Work out the finished part from the listing and answer in its coordinate system (mm). Coordinates: 2 decimals unless noted, no trailing zeros. Order: outer loops, then holes, each group sorted by start corner. A loop starts at its lowest first (then second) coordinate and runs counter-clockwise, first axis right, second up. Notation, with made-up numbers: M -12.75,-36.5 L 35.25,-36.5 A22 cw 35.25,1.5 Z; hole C 10.25,12 d6. An arc over 180 degrees is marked long. Answer in a Markdown table with one row per item. Add a question column.
Item 1: Consider line 1 (Z direction, x = 127.5, y = 1.75); line 2 (X direction, y = 3.9, z = 13); line 3 (Z direction, x = 57, y = 4.55). Determine where each line is inside the solid, lowest interval first. Write a range as from..to.
Item 2: The part is cut by section C-C (z = 33). Write down the section's boundary in (x, y), then the cut area to 3 significant figures.
Item 3: The part is cut by section A-A (z = 7). Write down the section's boundary in (x, y), then the cut area to 3 significant figures.
Item 4: The part is cut by section D-D (x = 19). Write down the section's boundary in (y, z), then the cut area to 3 significant figures.
Item 5: The part is cut by section B-B (x = 51). Write down the section's boundary in (y, z).
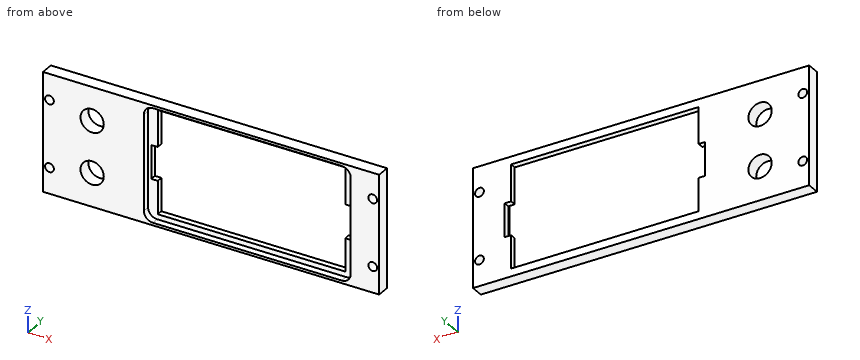
Autodesk Fusion 360 part; units mm, degrees
sketch "Sketch1" plane through (0, 0, 0) normal (0, 0, 1) x (1, 0, 0)
  line L0 (0, 0) -> (130, 0)
  line L1 (130, 0) -> (130, 5)
  line L2 (130, 5) -> (0, 5)
  line L3 (0, 5) -> (0, 0)
  dimension "d1" = 130
  dimension "d2" = 5
extrude "Extrude1" add sketch "Sketch1" along normal blind 46
sketch "Sketch2" plane through (0, 0, 0) normal (0, -1, 0) x (1, 0, 0)
  line L0 (0, 0) -> (130, 0)
  line L1 (130, 0) -> (130, 46)
  line L2 (130, 46) -> (0, 46)
  line L3 (0, 46) -> (0, 0)
  line L4 (42.5, 45) -> (115.5, 45)
  line L5 (119, 41.5) -> (119, 4.5)
  line L6 (115.5, 1) -> (42.5, 1)
  line L7 (39, 4.5) -> (39, 41.5)
  line L8 (125, 46) -> (125, 0) construction
  line L9 (5, 46) -> (5, 0) construction
  line L10 (42.75, 43) -> (115.25, 43)
  line L11 (115.25, 3) -> (42.75, 3)
  line L12 (42.75, 28.8154) -> (40.25, 28.8154)
  line L13 (40.25, 28.8154) -> (40.25, 15.8154)
  line L14 (40.25, 15.8154) -> (42.75, 15.8154)
  line L15 (115.25, 28.8154) -> (117.75, 28.8154)
  line L16 (117.75, 28.8154) -> (117.75, 15.8154)
  line L17 (117.75, 15.8154) -> (115.25, 15.8154)
  line L18 (115.25, 43) -> (115.25, 28.8154)
  line L19 (115.25, 15.8154) -> (115.25, 3)
  line L20 (42.75, 3) -> (42.75, 15.8154)
  line L21 (42.75, 28.8154) -> (42.75, 43)
  arc A0 (42.5, 45) -> (39, 41.5) centre (42.5, 41.5) ccw
  arc A1 (119, 41.5) -> (115.5, 45) centre (115.5, 41.5) ccw
  arc A2 (115.5, 1) -> (119, 4.5) centre (115.5, 4.5) ccw
  arc A3 (39, 4.5) -> (42.5, 1) centre (42.5, 4.5) ccw
  point P0 (39, 45)
  point P1 (119, 45)
  point P2 (39, 1)
  dimension "d5" = 80
  dimension "d6" = 44
  dimension "d7" = 5
  dimension "d8" = 5
  dimension "d9" = 6
  dimension "d10" = 1
  dimension "d25" = 2.5
  dimension "d26" = 13
  dimension "d28" = 13
  dimension "d35" = 3.5
  dimension "d59" = 72.5
  dimension "d60" = 40
  dimension "d62" = 2.5
  dimension "d63" = 1.25
  dimension "d64" = 2
extrude "Extrude5" cut sketch "Sketch2" against normal blind 5 contours L10 L11 L12 L13 L14 L15 L16 L17 L18 L19 L20 L21
sketch "Sketch4" plane through (0, 5, 0) normal (0, 1, 0) x (-1, 0, 0)
  line L0 (-40.25, 15.8154) -> (-42.75, 15.8154)
  line L1 (-42.75, 15.8154) -> (-42.75, 3)
  line L2 (-42.75, 3) -> (-115.25, 3)
  line L3 (-115.25, 3) -> (-115.25, 15.8154)
  line L4 (-115.25, 15.8154) -> (-117.75, 15.8154)
  line L5 (-117.75, 15.8154) -> (-117.75, 28.8154)
  line L6 (-117.75, 28.8154) -> (-115.25, 28.8154)
  line L7 (-115.25, 28.8154) -> (-115.25, 43)
  line L8 (-115.25, 43) -> (-42.75, 43)
  line L9 (-42.75, 43) -> (-42.75, 28.8154)
  line L10 (-42.75, 28.8154) -> (-40.25, 28.8154)
  line L11 (-40.25, 28.8154) -> (-40.25, 15.8154)
  line L12 (-130, 0) -> (0, 0)
  line L13 (0, 0) -> (0, 46)
  line L14 (0, 46) -> (-130, 46)
  line L15 (-130, 46) -> (-130, 0)
  line L16 (-118.25, 45) -> (-39.25, 45)
  line L17 (-39.25, 45) -> (-39.25, 2)
  line L18 (-39.25, 2) -> (-118.25, 2)
  line L19 (-118.25, 2) -> (-118.25, 45)
  line L20 (-42.75, 43) -> (-115.25, 43)
  dimension "d31" = 79
  dimension "d32" = 43
  dimension "d33" = 2
  dimension "d34" = 3.5
extrude "Extrude6" cut sketch "Sketch2" against normal blind 2.7 contours L4 L5 L6 L7 A0 A1 A2 A3
sketch "Sketch5" plane through (0, 0, 0) normal (0, -1, 0) x (1, 0, 0)
  line L0 (39, 4.5) -> (39, 41.5)
  arc A0 (42.5, 45) -> (39, 41.5) centre (42.5, 41.5) ccw
  line L1 (42.5, 45) -> (115.5, 45)
  arc A1 (119, 41.5) -> (115.5, 45) centre (115.5, 41.5) ccw
  line L2 (119, 41.5) -> (119, 4.5)
  arc A2 (115.5, 1) -> (119, 4.5) centre (115.5, 4.5) ccw
  line L3 (115.5, 1) -> (42.5, 1)
  arc A3 (39, 4.5) -> (42.5, 1) centre (42.5, 4.5) ccw
  line L4 (0, 0) -> (130, 0)
  line L5 (130, 0) -> (130, 46)
  line L6 (130, 46) -> (0, 46)
  line L7 (0, 46) -> (0, 0)
  line L8 (19, 33) -> (19, 13) construction
  line L9 (5, 46) -> (5, 0) construction
  line L10 (39, 23) -> (19, 23) construction
  point P0 (19, 33)
  point P1 (19, 13)
  point P2 (19, 33)
  point P3 (19, 33)
  point P4 (19, 33)
  point P5 (19, 13)
  dimension "d40" = 20
  dimension "d41" = 20
  dimension "d42" = 5
hole "Hole1" at (19, 0, 33) at (19, 0, 13) direction (0, 1, 0) diameter 9 end through all
sketch "Sketch6" plane through (0, 0, 0) normal (0, -1, 0) x (1, 0, 0)
  circle A0 centre (19, 33) radius 4.5
  circle A1 centre (19, 13) radius 4.5
  line L0 (39, 4.5) -> (39, 41.5)
  arc A2 (42.5, 45) -> (39, 41.5) centre (42.5, 41.5) ccw
  line L1 (42.5, 45) -> (115.5, 45)
  arc A3 (119, 41.5) -> (115.5, 45) centre (115.5, 41.5) ccw
  line L2 (119, 41.5) -> (119, 4.5)
  arc A4 (115.5, 1) -> (119, 4.5) centre (115.5, 4.5) ccw
  line L3 (115.5, 1) -> (42.5, 1)
  arc A5 (39, 4.5) -> (42.5, 1) centre (42.5, 4.5) ccw
  line L4 (0, 0) -> (130, 0)
  line L5 (130, 0) -> (130, 46)
  line L6 (130, 46) -> (0, 46)
  line L7 (0, 46) -> (0, 0)
  line L8 (125, 46) -> (125, 0) construction
  line L9 (5, 46) -> (5, 0) construction
  point P0 (2.5, 36)
  point P1 (2.5, 10)
  point P2 (127.5, 36)
  point P3 (127.5, 10)
  dimension "d46" = 5
  dimension "d47" = 5
  dimension "d48" = 2.5
  dimension "d49" = 10
  dimension "d50" = 10
  dimension "d51" = 2.5
  dimension "d52" = 2.5
  dimension "d53" = 10
  dimension "d54" = 10
  dimension "d55" = 2.5
hole "Hole2" at (127.5, 0, 36) at (127.5, 0, 10) at (2.5, 0, 36) at (2.5, 0, 10) direction (0, 1, 0) diameter 3.4 depth 5 tip angle 180
Reply:
| question | item | result |
|---|---|---|
| 1 | line 1 | z = 0..8.3, 11.7..34.3, 37.7..46 |
| 1 | line 2 | x = 0..14.5, 23.5..42.75, 115.25..130 |
| 1 | line 3 | z = 0..3, 43..46 |
| 2 | outline | M 0,0 L 14.5,0 L 14.5,5 L 0,5 Z; M 23.5,0 L 39,0 L 39,2.7 L 42.75,2.7 L 42.75,5 L 23.5,5 Z; M 115.25,2.7 L 119,2.7 L 119,0 L 130,0 L 130,5 L 115.25,5 Z |
| 2 | area | 222 mm2 |
| 3 | outline | M 0,0 L 39,0 L 39,2.7 L 42.75,2.7 L 42.75,5 L 0,5 Z; M 115.25,2.7 L 119,2.7 L 119,0 L 130,0 L 130,5 L 115.25,5 Z |
| 3 | area | 267 mm2 |
| 4 | outline | M 0,0 L 5,0 L 5,8.5 L 0,8.5 Z; M 0,17.5 L 5,17.5 L 5,28.5 L 0,28.5 Z; M 0,37.5 L 5,37.5 L 5,46 L 0,46 Z |
| 4 | area | 140 mm2 |
| 5 | outline | M 0,0 L 5,0 L 5,3 L 2.7,3 L 2.7,1 L 0,1 Z; M 0,45 L 2.7,45 L 2.7,43 L 5,43 L 5,46 L 0,46 Z |
